Verification items for the finished model (mm, model axes). A direction names the side the tool comes from. Give positions to 0.01 mm unless a question says otherwise; leave off trailing zeros. Write each loop counter-clockwise with the first axis right and the second up, starting at its lowest first coordinate (ties: lowest second). Pieces come first, ordered by that corner, then holes. Notation, with made-up numbers: (49.5, -14.5) -> (71.5, -14.5) arc R20 cw to (71.5, -10.5) -> close; hole circle Ø10 at (-15, 28.25). An arc over 180 degrees is marked (long way). Write item = value, one per line.
from build123d import *

# Parameters (mm, degrees)
ESQUISSE1_R                  = 4.25
ESQUISSE1_R_2                = 1.5
BOSS_EXTRU_1_DEPTH           = 5
ESQUISSE2_R                  = 3
ENL_V_MAT_EXTRU_1_DEPTH      = 3
BOSS_EXTRU_2_DEPTH           = 3
R_P_TITION_CIRCULAIRE1_DEPTH = 3
ESQUISSE4_R                  = 0.75
BOSS_EXTRU_3_DEPTH           = 2
R_P_TITION_CIRCULAIRE2_COUNT = 6
ENL_V_START                  = -1
ESQUISSE5_R                  = 3
ENL_V_MAT_EXTRU_2_DEPTH      = 1
CONG_1_R                     = 0.2
ESQUISSE6_R                  = 4.5
ESQUISSE6_R_2                = 3.5
ENL_V_MAT_EXTRU_3_DEPTH      = 1
CONG_2_R                     = 0.25


# Read off the part's stored shape, not the designer's step: Répétition circulaire1
with BuildPart() as part:
    # Esquisse1 → Boss.-Extru.1 (new body)
    with BuildSketch(Plane.XY):
        Circle(ESQUISSE1_R)
        Circle(ESQUISSE1_R_2, mode=Mode.SUBTRACT)
    extrude(amount=BOSS_EXTRU_1_DEPTH)

    # Esquisse2 → Enlèv. mat.-Extru.1 (cut)
    with BuildSketch(Plane(origin=(0, 0, 0), x_dir=(-1, 0, 0), z_dir=(0, 0, -1))):
        Circle(ESQUISSE2_R)
    extrude(amount=-ENL_V_MAT_EXTRU_1_DEPTH, mode=Mode.SUBTRACT)

    # Esquisse3 → Boss.-Extru.2 (add)
    with BuildSketch(Plane(origin=(0, 0, 0), x_dir=(-1, 0, 0), z_dir=(0, 0, -1))):
        Polygon((-0.3, 3), (0, 2.6), (0.3, 3), align=None)
    extrude(amount=-BOSS_EXTRU_2_DEPTH)

    # Répétition circulaire1 outline → Répétition circulaire1 (add)
    with BuildSketch(Plane.XY):
        with BuildLine():
            ThreePointArc((1.052468236, 2.80932565), (0.776457135, 2.897777479), (0.493198596, 2.959181499))
            Line((0.493198596, 2.959181499), (0.672929517, 2.511407148))
            Line((0.672929517, 2.511407148), (1.052468236, 2.80932565))
        make_face()
        with BuildLine():
            ThreePointArc((-0.493198596, 2.959181499), (-0.776457135, 2.897777479), (-1.052468236, 2.80932565))
            Line((-1.052468236, 2.80932565), (-0.672929517, 2.511407148))
            Line((-0.672929517, 2.511407148), (-0.493198596, 2.959181499))
        make_face()
        with BuildLine():
            ThreePointArc((-1.242285791, 2.730700645), (-1.5, 2.598076211), (-1.743713233, 2.441201376))
            Line((-1.743713233, 2.441201376), (-1.3, 2.25166605))
            Line((-1.3, 2.25166605), (-1.242285791, 2.730700645))
        make_face()
        with BuildLine():
            ThreePointArc((-1.906713263, 2.316127054), (-2.121320343, 2.121320343), (-2.316127054, 1.906713263))
            Line((-2.316127054, 1.906713263), (-1.838477631, 1.838477631))
            Line((-1.838477631, 1.838477631), (-1.906713263, 2.316127054))
        make_face()
        with BuildLine():
            ThreePointArc((-2.441201376, 1.743713233), (-2.598076211, 1.5), (-2.730700645, 1.242285791))
            Line((-2.730700645, 1.242285791), (-2.25166605, 1.3))
            Line((-2.25166605, 1.3), (-2.441201376, 1.743713233))
        make_face()
        with BuildLine():
            ThreePointArc((-2.809325651, 1.052468236), (-2.897777479, 0.776457135), (-2.959181499, 0.493198596))
            Line((-2.959181499, 0.493198596), (-2.511407148, 0.672929517))
            Line((-2.511407148, 0.672929517), (-2.809325651, 1.052468236))
        make_face()
        with BuildLine():
            ThreePointArc((-2.985999024, 0.289499268), (-3, 0), (-2.985999024, -0.289499268))
            Line((-2.985999024, -0.289499268), (-2.6, 0))
            Line((-2.6, 0), (-2.985999024, 0.289499268))
        make_face()
        with BuildLine():
            ThreePointArc((-2.959181499, -0.493198596), (-2.897777479, -0.776457135), (-2.809325651, -1.052468236))
            Line((-2.809325651, -1.052468236), (-2.511407148, -0.672929517))
            Line((-2.511407148, -0.672929517), (-2.959181499, -0.493198596))
        make_face()
        with BuildLine():
            ThreePointArc((-2.730700645, -1.242285791), (-2.598076211, -1.5), (-2.441201377, -1.743713233))
            Line((-2.441201377, -1.743713233), (-2.25166605, -1.3))
            Line((-2.25166605, -1.3), (-2.730700645, -1.242285791))
        make_face()
        with BuildLine():
            ThreePointArc((-2.316127055, -1.906713263), (-2.121320344, -2.121320344), (-1.906713263, -2.316127055))
            Line((-1.906713263, -2.316127055), (-1.838477631, -1.838477631))
            Line((-1.838477631, -1.838477631), (-2.316127055, -1.906713263))
        make_face()
        with BuildLine():
            ThreePointArc((-1.743713233, -2.441201377), (-1.5, -2.598076211), (-1.242285791, -2.730700645))
            Line((-1.242285791, -2.730700645), (-1.3, -2.25166605))
            Line((-1.3, -2.25166605), (-1.743713233, -2.441201377))
        make_face()
        with BuildLine():
            ThreePointArc((-1.052468236, -2.809325651), (-0.776457135, -2.897777479), (-0.493198596, -2.959181499))
            Line((-0.493198596, -2.959181499), (-0.672929517, -2.511407148))
            Line((-0.672929517, -2.511407148), (-1.052468236, -2.809325651))
        make_face()
        with BuildLine():
            ThreePointArc((-0.289499268, -2.985999024), (0, -3), (0.289499268, -2.985999024))
            Line((0.289499268, -2.985999024), (0, -2.6))
            Line((0, -2.6), (-0.289499268, -2.985999024))
        make_face()
        with BuildLine():
            ThreePointArc((0.493198596, -2.959181499), (0.776457135, -2.897777479), (1.052468236, -2.809325651))
            Line((1.052468236, -2.809325651), (0.672929517, -2.511407148))
            Line((0.672929517, -2.511407148), (0.493198596, -2.959181499))
        make_face()
        with BuildLine():
            ThreePointArc((1.242285791, -2.730700645), (1.5, -2.598076211), (1.743713233, -2.441201377))
            Line((1.743713233, -2.441201377), (1.3, -2.25166605))
            Line((1.3, -2.25166605), (1.242285791, -2.730700645))
        make_face()
        with BuildLine():
            ThreePointArc((1.906713263, -2.316127055), (2.121320344, -2.121320344), (2.316127055, -1.906713263))
            Line((2.316127055, -1.906713263), (1.838477631, -1.838477631))
            Line((1.838477631, -1.838477631), (1.906713263, -2.316127055))
        make_face()
        with BuildLine():
            ThreePointArc((2.441201377, -1.743713233), (2.598076211, -1.5), (2.730700645, -1.242285791))
            Line((2.730700645, -1.242285791), (2.25166605, -1.3))
            Line((2.25166605, -1.3), (2.441201377, -1.743713233))
        make_face()
        with BuildLine():
            ThreePointArc((2.809325651, -1.052468236), (2.897777479, -0.776457135), (2.959181499, -0.493198596))
            Line((2.959181499, -0.493198596), (2.511407148, -0.672929517))
            Line((2.511407148, -0.672929517), (2.809325651, -1.052468236))
        make_face()
        with BuildLine():
            ThreePointArc((2.985999024, -0.289499268), (3, 0), (2.985999024, 0.289499268))
            Line((2.985999024, 0.289499268), (2.6, 0))
            Line((2.6, 0), (2.985999024, -0.289499268))
        make_face()
        with BuildLine():
            ThreePointArc((2.959181499, 0.493198596), (2.897777479, 0.776457135), (2.809325651, 1.052468236))
            Line((2.809325651, 1.052468236), (2.511407148, 0.672929517))
            Line((2.511407148, 0.672929517), (2.959181499, 0.493198596))
        make_face()
        with BuildLine():
            ThreePointArc((2.730700645, 1.242285791), (2.598076211, 1.5), (2.441201376, 1.743713233))
            Line((2.441201376, 1.743713233), (2.25166605, 1.3))
            Line((2.25166605, 1.3), (2.730700645, 1.242285791))
        make_face()
        with BuildLine():
            ThreePointArc((2.316127054, 1.906713263), (2.121320343, 2.121320343), (1.906713263, 2.316127054))
            Line((1.906713263, 2.316127054), (1.838477631, 1.838477631))
            Line((1.838477631, 1.838477631), (2.316127054, 1.906713263))
        make_face()
        with BuildLine():
            ThreePointArc((1.743713233, 2.441201376), (1.5, 2.598076211), (1.242285791, 2.730700645))
            Line((1.242285791, 2.730700645), (1.3, 2.25166605))
            Line((1.3, 2.25166605), (1.743713233, 2.441201376))
        make_face()
    extrude(amount=R_P_TITION_CIRCULAIRE1_DEPTH)

    # Esquisse4 → Boss.-Extru.3 (add)
    with BuildSketch(Plane.XY.offset(5)):
        with BuildLine():
            Line((-1.95061736, 14.441692106), (-3.75, 6.495190528))
            Line((-3.75, 6.495190528), (-3.75, 2))
            Line((-3.75, 2), (0, 3.364888378))
            Line((0, 3.364888378), (3.75, 2))
            Line((3.75, 2), (3.75, 6.495190528))
            Line((3.75, 6.495190528), (1.95061736, 14.441692106))
            ThreePointArc((1.95061736, 14.441692106), (0, 16), (-1.95061736, 14.441692106))
        make_face()
        with Locations((0, 7.5)):
            Circle(ESQUISSE4_R, mode=Mode.SUBTRACT)
        with Locations((0, 10.5)):
            Circle(ESQUISSE4_R, mode=Mode.SUBTRACT)
        with Locations((0, 13.5)):
            Circle(ESQUISSE4_R, mode=Mode.SUBTRACT)
    boss_extru_3 = extrude(amount=-BOSS_EXTRU_3_DEPTH)

    # Répétition circulaire2: Boss.-Extru.3 ×6 about axis
    r_p_tition_circulaire2_axis = Axis((0, 0, 0), (0, 0, 1))
    for i in range(1, R_P_TITION_CIRCULAIRE2_COUNT):
        add(boss_extru_3.rotate(r_p_tition_circulaire2_axis, i * 360 / R_P_TITION_CIRCULAIRE2_COUNT))

    # Esquisse5 → Enlèv. mat.-Extru.2 (cut)
    with BuildSketch(Plane.XY.offset(5).offset(ENL_V_START)):
        Circle(ESQUISSE5_R)
    extrude(amount=ENL_V_MAT_EXTRU_2_DEPTH, mode=Mode.SUBTRACT)

    # Congé1
    cong_1_edges = [part.edges().sort_by_distance(p)[0] for p in [
        (-4.25, 0, 0),
    ]]
    fillet(cong_1_edges, radius=CONG_1_R)

    # Esquisse6 → Enlèv. mat.-Extru.3 (cut)
    with BuildSketch(Plane.XY.offset(5)):
        Circle(ESQUISSE6_R)
        Circle(ESQUISSE6_R_2, mode=Mode.SUBTRACT)
    extrude(amount=-ENL_V_MAT_EXTRU_3_DEPTH, mode=Mode.SUBTRACT)

    # Congé2
    cong_2_edges = [part.edges().sort_by_distance(p)[0] for p in [
        (-3, 0, 5),
        (-4.5, 0, 5),
        (-3.5, 0, 5),
    ]]
    fillet(cong_2_edges, radius=CONG_2_R - 0.0001)  # a hair under: the kernel refuses the full size


solid = part.part
Item 1: Sectioned sample at C-C on y = 12. Record the cut outline in (x, z), then the cut area to 3 significant figures.
Response values:
outline = (-2.5, 3) -> (2.5, 3) -> (2.5, 5) -> (-2.5, 5) -> close
area = 10.0 mm^2
Item 2: Set-up check for faces 1 (the flat face through (-7.7, -7.72, 4.01)), 2 (the flat face through (1.3, -1.3, 4)), 3 (the flat face through (-10.53, 2.8, 4.01)): record each of +Z, -Z, +X, -X, +Y, -Y from which the full face is reachable in a straight line by a thin tool's end or side.
Response values:
face_1 = +Z, -Z, -Y
face_2 = +Z
face_3 = +Z, -Z, -X
Item 3: Go/stop test with flat-tipped pins: P1, Ø10, axis at x = 8, y = 8, coming from the -Z side; P2, Ø2.5, axis at x = -1, y = 0.5, coming from the +Z side; P3, Ø3, axis at x = -5, z = 2, coming from the -Y side. Record where each tip stops, or that it passes through.
Response values:
P1 = 3
P2 = 4
P3 = -7.23
Item 4: Mould release check, pull along Y, two halves, no side actions. Record for faces 4 (the cylindrical face through (0, -16, 4)), 5 (the flat face through (-2.84, 10.52, 4.01)), 6 (the cylindrical face through (-0.59, 4.46, 4.38)), 7 (the cylindrical face through (11, 7.04, 4.01)): +Y half, -Y half, draft (parallel to the pull), parting line (faces both ways), or undercut.
Response values:
face_4 = -Y half
face_5 = +Y half
face_6 = undercut
face_7 = undercut
Item 5: Sectioned sample at B-B on z = 3.6. Give the number of separate pieces and of enclosed holes in the cut face, then the cut area to 3 significant figures.
Response values:
separate_pieces = 1
enclosed_holes = 19
area = 406 mm^2
Item 6: Sectioned sample at A-A on x = -10.25. Record the cut outline in (y, z).
Response values:
outline = (-8.51, 3) -> (-2.54, 3) -> (-2.54, 5) -> (-8.51, 5) -> close; (2.54, 3) -> (8.51, 3) -> (8.51, 5) -> (2.54, 5) -> close
Item 7: Material ranges on line 1 (Y direction, x = 9.5, z = 3.7); line 2 (Z direction, x = -0.5, y = 3.5); line 3 (Z direction, x = -1.75, y = -0.5), recorded low to high.
Response values:
line_1 = -8.28 to -5.88, -4.62 to -1.85, 1.85 to 4.62, 5.88 to 8.28
line_2 = 0 to 4
line_3 = 3 to 4
